Geometry: see drawing. Coordinates: mm, zero at the bounding-box minimum. Coordinates: 2 decimals unless noted, no trailing zeros. Order: outer loops, then holes, each group sorted by start corner. A loop starts at its lowest first (then second) coordinate and runs counter-clockwise, first axis right, second up. Notation, with made-up numbers: (-12.5, -12.75) -> (35.5, -12.75) arc R12 ccw to (35.5, 9.25) -> close; hole circle Ø5 at (22.5, 87.5). An arc over 180 degrees is marked (long way). Use one line per item in the form item = value.
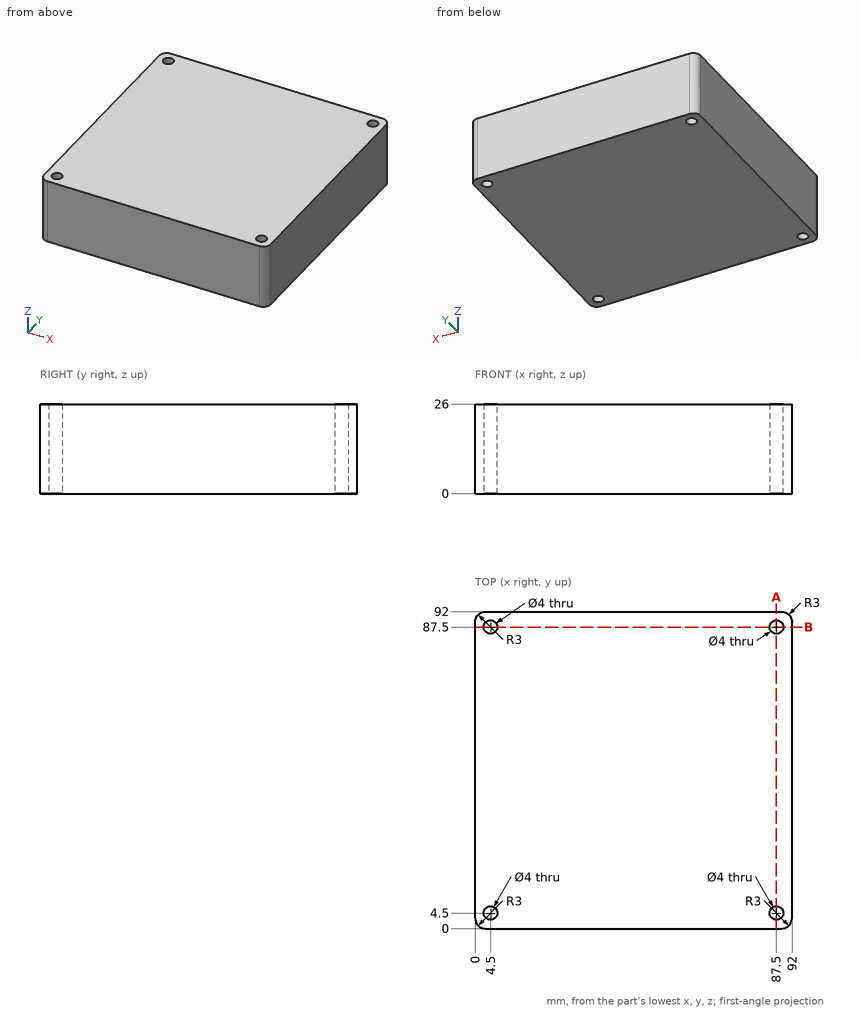
1) Section A-A, the plane x = 87.5. Output: boundary loops of the cut face in (y, z), and give its area (3 significant figures).
Results found:
outline = (0, 0) -> (2.5, 0) -> (2.5, 26) -> (0, 26) -> close; (6.5, 0) -> (85.5, 0) -> (85.5, 26) -> (6.5, 26) -> close; (89.5, 0) -> (92, 0) -> (92, 26) -> (89.5, 26) -> close
area = 2,180 mm2
2) Material intervals for probe 1 along Y at (x, z) = (87.5, 13.5); probe 2 along X at (y, z) = (5, 4.75), sorted ascending. Write a range as from..to.
Results found:
probe_1 = 0..2.5, 6.5..85.5, 89.5..92
probe_2 = 0..2.56, 6.44..85.56, 89.44..92
